CAD build for the part. Positions are in the model's coordinates, mm. A direction names the side the tool comes from. Round coordinates to 2 decimals unless told otherwise and drop trailing zeros. Order: outer loops, then holes, each group sorted by start corner. A loop starts at its lowest first (then second) coordinate and runs counter-clockwise, first axis right, second up. Notation, with made-up numbers: M 82,81.25 L 104,81.25 A30 ccw 104,119.25 Z; hole C 23.5,20 d10. An arc over 180 degrees is marked long. Answer as a JSON object with one key per item and string values.
```python
from build123d import *

# Parameters (mm, degrees)
F0_W     = 56
F0_H     = 116
F1_DEPTH = 5
F2_R     = 8
F3_R     = 1.75
F4_DEPTH = 13
F5_W     = 9.9999913867
F5_H     = 3
F6_DEPTH = 0.3


with BuildPart() as f1:
    # F0 (on Front) → F1 (new body, symmetric)
    with BuildSketch(Plane.XZ):
        Rectangle(F0_W, F0_H)
    extrude(amount=F1_DEPTH, both=True)

    # F2
    f2_edges = [f1.edges().sort_by_distance(p)[0] for p in [
        (-28, 0, 58),
        (28, 0, 58),
        (28, 0, -58),
        (-28, 0, -58),
    ]]
    fillet(f2_edges, radius=F2_R)

    # F3 (on face) → F4 (cut)
    with BuildSketch(Plane.XY.offset(58)):
        with Locations((-15.25, 0)):
            Circle(F3_R)
    extrude(amount=-F4_DEPTH, mode=Mode.SUBTRACT)

    # F5 (on face) → F6 (join)
    with BuildSketch(Plane.XY.offset(58)):
        with Locations((11.5000043066, 0)):
            Rectangle(F5_W, F5_H)
        with BuildLine():
            Line((6.5000086133, -1.5), (6.5000086133, 1.5))
            ThreePointArc((6.5000086133, 1.5), (5.0000086133, 0), (6.5000086133, -1.5))
        make_face()
        with BuildLine():
            ThreePointArc((16.5, -1.5), (18, 0), (16.5, 1.5))
            Line((16.5, 1.5), (16.5, -1.5))
        make_face()
    extrude(amount=F6_DEPTH)


solid = f1.part
```
Item 1: 3-axis set-ups, long thin cutter, end or side, ignore diameter. For faces 1 (the cylindrical face through (25.719, -0.07, -55.594)), 2 (the cylindrical face through (-13.581, 0.526, 51.591)): which of +Z, -Z, +X, -X, +Y, -Y reach the whole face in a straight line?
Worked answers:
{"face 1": "-Z, +X, +Y, -Y", "face 2": "+Z"}
Item 2: Drop flat-ended pins along their axis: pin 1 Ø3 at (x, y) = (-15.25, 0) entering from +Z; pin 2 Ø5 at (x, y) = (-9, 1) entering from +Z; pin 3 Ø4 at (x, y) = (3.5, 0) entering from +Z. Give the stop position or say it passes through.
Worked answers:
{"pin 1": "stops at z = 45", "pin 2": "stops at z = 58", "pin 3": "stops at z = 58.3"}
Item 3: Wall check: line 1 along Y through (x, z) = (-15, 50); line 2 along Z through (x, y) = (-12, 2.25); line 3 along Z through (x, y) = (25.5, -2.75). Give the ranges that are in metal, low to high. Write a range as [from, to].
Worked answers:
{"line 1": "y = [-5, -1.73], [1.73, 5]", "line 2": "z = [-58, 58]", "line 3": "z = [-55.81, 55.81]"}
Item 4: Saw through at C-C on x = -15.25. List the corners of the cut face in (y, z).
Worked answers:
{"outline": "M -5,-58 L 5,-58 L 5,58 L 1.75,58 L 1.75,45 L -1.75,45 L -1.75,58 L -5,58 Z"}
Item 5: Saw through at B-B on z = 47.5. List the corners of the cut face in (x, y), and give its area (3 significant figures).
Worked answers:
{"outline": "M -28,-5 L 28,-5 L 28,5 L -28,5 Z; hole C -15.25,0 d3.5", "area": "550 mm2"}
Item 6: Two-plate mould, pull along Y, no slides. Class faces 3 (the flat face through (0, 0, -58)), 4 (the flat face through (-15, 0, 45)), 5 (the flat face through (0, -5, 1)): released by +Y, released by -Y, zero draft, split by the parting line, or undercut.
Worked answers:
{"face 3": "zero draft", "face 4": "undercut", "face 5": "released by -Y"}
Item 7: Saw through at A-A on y = 0. List the corners of the cut face in (x, z), and give its area (3 significant figures).
Worked answers:
{"outline": "M -28,-50 A8 ccw -20,-58 L 20,-58 A8 ccw 28,-50 L 28,50 A8 ccw 20,58 L 18,58 L 18,58.3 L 5,58.3 L 5,58 L -13.5,58 L -13.5,45 L -17,45 L -17,58 L -20,58 A8 ccw -28,50 Z", "area": "6,400 mm2"}
